from build123d import *

# Parameters (mm, degrees)
BOSS_EXTRUDE1_DEPTH       = 4.7625
F_4_CLEARANCE_HOLE1_D     = 3.2639
F_4_CLEARANCE_HOLE1_DEPTH = 12.7
F_4_CLEARANCE_HOLE1_TIP   = 0.980574487
FILLET1_R                 = 4.7625
FILLET2_R                 = 6.35


with BuildPart() as part:
    # Sketch1 → Boss-Extrude1 (new, symmetric)
    with BuildSketch(Plane.XY):
        Polygon((0, 0), (0, -47.625), (95.25, 0), align=None)
    extrude(amount=BOSS_EXTRUDE1_DEPTH, both=True)

    # #4 Clearance Hole1
    with Locations(Plane.XY.offset(4.7625)):
        with Locations((7.9375, -7.9375), (63.5, -7.9375), (7.9375, -33.3375)):
            Hole(F_4_CLEARANCE_HOLE1_D / 2, depth=F_4_CLEARANCE_HOLE1_DEPTH)
            with Locations((0, 0, -(F_4_CLEARANCE_HOLE1_DEPTH + F_4_CLEARANCE_HOLE1_TIP / 2))):  # 118° drill point
                Cone(0, F_4_CLEARANCE_HOLE1_D / 2, F_4_CLEARANCE_HOLE1_TIP, mode=Mode.SUBTRACT)

    # Fillet1
    fillet1_edges = [part.edges().sort_by_distance(p)[0] for p in [
        (0, -47.625, 0),
        (0, 0, 0),
    ]]
    fillet(fillet1_edges, radius=FILLET1_R)

    # Fillet2
    fillet2_edges = [part.edges().sort_by_distance(p)[0] for p in [
        (95.25, 0, 0),
    ]]
    fillet(fillet2_edges, radius=FILLET2_R)


solid = part.part
The model under review builds one solid part; all positions refer to its coordinate system, in mm. Round coordinates to 2 decimals unless told otherwise and drop trailing zeros. Order: outer loops, then holes, each group sorted by start corner. A loop starts at its lowest first (then second) coordinate and runs counter-clockwise, first axis right, second up. Notation, with made-up numbers: (66, 29.5) -> (123, 29.5) arc R12 ccw to (123, 45.5) -> close; hole circle Ø10 at (47, -12). An arc over 180 degrees is marked (long way). Use CSV: the item, a comma, the result in double quotes. Start each with the question number.
(1) Consider section C-C on y = -16.5. Write out the cut boundary in (x, z).
(2) Wall thickness on probe 1 along X at (y, z) = (-7, 1); probe 2 along Y at (x, z) = (63.5, -0.5) (3 decimals); probe 3 along X at (y, z) = (-8, -4): over which ranges is each line inside the solid? List them lowest first. Write a range as from..to.
(3) Consider section D-D on x = 21. Write out the cut boundary in (y, z) (1 decimal), and give its area (3 significant figures).
(4) Consider section A-A on x = 63.5. Write out the cut boundary in (y, z) (1 decimal).
(5) Insertion check: pin 1 (4 mm diameter, centred on x = 7.94, y = -33.34, fed in from +Z); pin 2 (3 mm diameter, centred on y = -13.5, z = 4, fed in from +X). Each pin has a flat end and moves straight along its axis. Give the tip position at first contact, or say it passes through.
(6) Mouldability with a two-part tool opening along X and no side actions: class faces 1 (the face through (9.233, -8.931, -0.067)), 2 (the face through (1.36, -1.43, -0.07)), 3 (the face through (37, 0, 0)) as pulls with the +X half, pulls with the -X half, needs draft (parallel to the pull), parting line crosses it, or undercut.
(7) Consider section B-B on z = 0.25. State how many separate pieces and enclosed holes the cut face has, and give its area (3 significant figures).
Responses:
1,outline,"(0, -4.76) -> (62.25, -4.76) -> (62.25, 4.76) -> (0, 4.76) -> close"
2,probe 1,"0..6.6, 9.27..62.16, 64.84..74.67"
2,probe 2,"-15.875..-9.569, -6.306..0"
2,probe 3,"0..6.31, 9.57..61.87, 65.13..74.48"
3,outline,"(-37.1, -4.8) -> (0, -4.8) -> (0, 4.8) -> (-37.1, 4.8) -> close"
3,area,"354 mm²"
4,outline,"(-15.9, -4.8) -> (-9.6, -4.8) -> (-9.6, 4.8) -> (-15.9, 4.8) -> close; (-6.3, -4.8) -> (0, -4.8) -> (0, 4.8) -> (-6.3, 4.8) -> close"
5,pin 1,"z = 4.76"
5,pin 2,"x = 71.25"
6,face 1,"undercut"
6,face 2,"pulls with the -X half"
6,face 3,"needs draft"
7,separate pieces,"1"
7,enclosed holes,"3"
7,area,"2,110 mm²"
